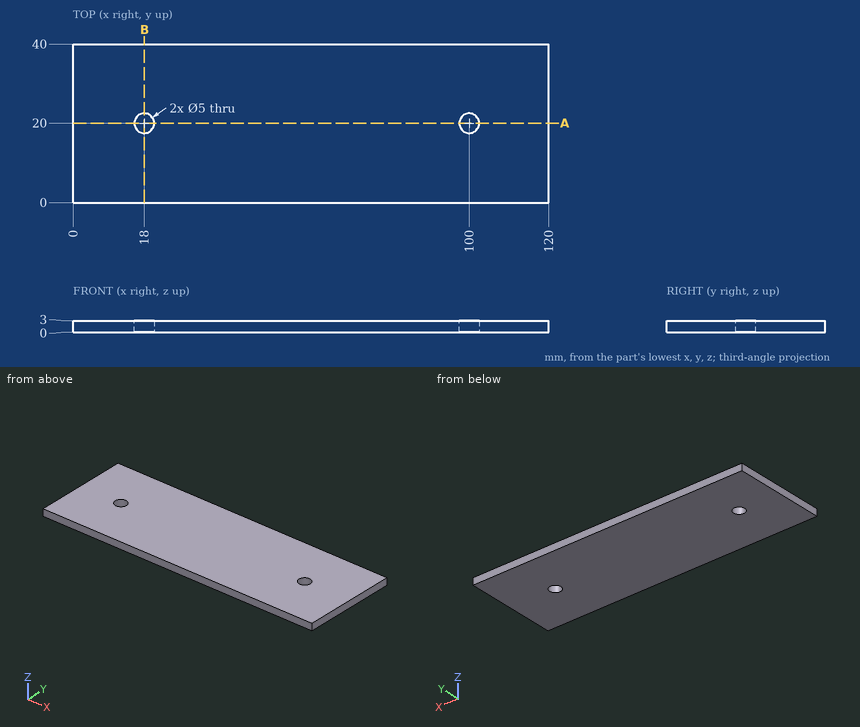
Input: dimensioned drawing with shaded views. Units: mm. Origin: part minimum x, y, z. Give positions to 0.01 mm unless a question says otherwise; leave off trailing zeros. Order: outer loops, then holes, each group sorted by start corner. A loop starts at its lowest first (then second) coordinate and runs counter-clockwise, first axis right, second up. Notation, with made-up numbers: (49.25, 3.25) -> (94.25, 3.25) arc R18 cw to (94.25, 20.25) -> close; hole circle Ø4 at (30, 67.25). An arc over 180 degrees is marked (long way). Write item = value, one per line.
Item 1: Ray query, probe 1 along Y at (x, z) = (18, 2.1); probe 2 along X at (y, z) = (20.5, 0.65); probe 3 along X at (y, z) = (19, 1.15). Return the intervals inside material, ascending.
Check result:
probe_1 = 0 to 17.5, 22.5 to 40
probe_2 = 0 to 15.55, 20.45 to 97.55, 102.45 to 120
probe_3 = 0 to 15.71, 20.29 to 97.71, 102.29 to 120
Item 2: Section query B-B (x = 18). Output: boundary loops of the cut face in (y, z), then the cut area to 3 significant figures.
Check result:
outline = (0, 0) -> (17.5, 0) -> (17.5, 3) -> (0, 3) -> close; (22.5, 0) -> (40, 0) -> (40, 3) -> (22.5, 3) -> close
area = 105 mm²
Item 3: Section query A-A (y = 20). Output: boundary loops of the cut face in (x, z).
Check result:
outline = (0, 0) -> (15.5, 0) -> (15.5, 3) -> (0, 3) -> close; (20.5, 0) -> (97.5, 0) -> (97.5, 3) -> (20.5, 3) -> close; (102.5, 0) -> (120, 0) -> (120, 3) -> (102.5, 3) -> close
